```python
from build123d import *

# Parameters (mm, degrees)
F3_W     = 660
F3_H     = 200
F4_DEPTH = 450
F5_T     = -3
F6_R     = 10
F7_R     = 10
F8_R     = 10


with BuildPart() as f4:
    # F3 (on Front) → F4 (new body)
    with BuildSketch(Plane.XZ):
        with Locations((0, -100)):
            Rectangle(F3_W, F3_H)
    extrude(amount=F4_DEPTH)

    # F5
    f5_openings = [f4.faces().sort_by_distance(p)[0] for p in [
        (0, -450, -100),
    ]]
    offset(amount=F5_T, openings=f5_openings)

    # F6
    f6_edges = [f4.edges().sort_by_distance(p)[0] for p in [
        (330, -225, -200),
        (330, -225, 0),
    ]]
    fillet(f6_edges, radius=F6_R)

    # F7
    f7_edges = [f4.edges().sort_by_distance(p)[0] for p in [
        (327, -226.5, -197),
        (327, -226.5, -3),
        (-327, -226.5, -197),
        (-327, -226.5, -3),
    ]]
    fillet(f7_edges, radius=F7_R)

    # F8
    f8_edges = [f4.edges().sort_by_distance(p)[0] for p in [
        (-330, -225, -200),
        (-330, -225, 0),
    ]]
    fillet(f8_edges, radius=F8_R)


solid = f4.part
```
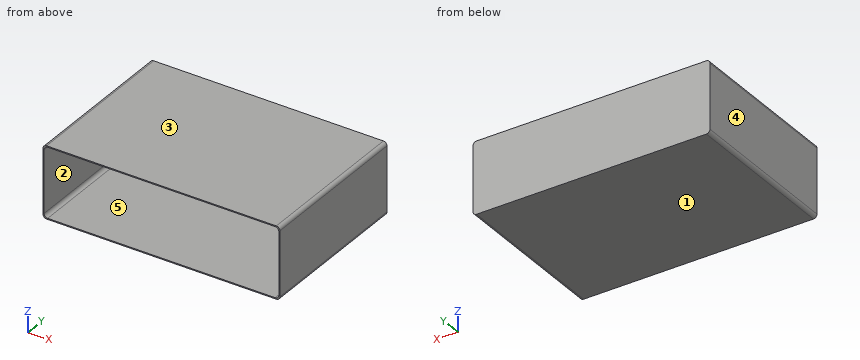
Input: part model. Units: mm. Frame: model coordinates. Face numbers are marked on the shaded views. A direction names the side the tool comes from. Coordinates: 2 decimals unless noted, no trailing zeros. Write each loop counter-clockwise with the first axis right and the second up, starting at its lowest first coordinate (ties: lowest second). Pieces come first, ordered by that corner, then holes. Notation, with made-up numbers: M 9.25,33.25 L 50.25,33.25 A33 ccw 50.25,64.25 Z; hole C 40,71 d3. An arc over 180 degrees is marked long. Use one line per item in the form item = value.
Q1. Draft query along X for the marked faces 3, 4 and 5. Return one class per face: released by +X, released by -X, zero draft, split by the parting line, or undercut.
Answer below:
face_3 = zero draft
face_4 = released by -X
face_5 = undercut
Q2. First-contact query: pin 1 (2 mm diameter, centred on x = 218, z = -154.5, fed in from -Y). Flat tip, straight axial feed; report the tip coordinate or a pass-through.
Answer below:
pin_1 = -3
Q3. Section C-C (z = -54.5). Return loops of the section in (x, y).
Answer below:
outline = M -330,-450 L -327,-450 L -327,-3 L 327,-3 L 327,-450 L 330,-450 L 330,0 L -330,0 Z
Q4. Section B-B (y = -111). Return loops of the section in (x, z), plus the area to 3 significant figures.
Answer below:
outline = M -330,-190 A10 ccw -320,-200 L 320,-200 A10 ccw 330,-190 L 330,-10 A10 ccw 320,0 L -320,0 A10 ccw -330,-10 Z; hole M -327,-187 A10 ccw -317,-197 L 317,-197 A10 ccw 327,-187 L 327,-13 A10 ccw 317,-3 L -317,-3 A10 ccw -327,-13 Z
area = 5,120 mm²
Q5. Set-up query: the marked faces 1 and 2. Return all of +Z, -Z, +X, -X, +Y, -Y with unobstructed straight access to the full face (end or side cutting, diameter ignored); none if empty.
Answer below:
face_1 = -Z, +X, -X, +Y, -Y
face_2 = -Y
Q6. Material intervals for probe 1 along Z at (x, y) = (-179, -321.5); probe 2 along X at (y, z) = (-348.5, -28.5); probe 3 along Y at (x, z) = (68, -33.5), sorted ascending. Write a range as from..to.
Answer below:
probe_1 = -200..-197, -3..0
probe_2 = -330..-327, 327..330
probe_3 = -3..0
Q7. Section A-A (x = -102). Return loops of the section in (y, z).
Answer below:
outline = M -450,-200 L 0,-200 L 0,0 L -450,0 L -450,-3 L -3,-3 L -3,-197 L -450,-197 Z
